Answer from the drawing. Dimensions are ordinates in mm from the lowest x, y and z of the part. Coordinates: 2 decimals unless noted, no trailing zeros. Write each loop counter-clockwise with the first axis right and the second up, starting at its lowest first coordinate (ties: lowest second). Pieces come first, ordered by that corner, then holes. Notation, with made-up numbers: (-37.5, -24.75) -> (19.5, -24.75) arc R18 ccw to (19.5, -10.75) -> close; hole circle Ø7 at (-26, -9.5). An arc over 180 degrees is marked (long way). Return JSON: item names as keys, results as strings.
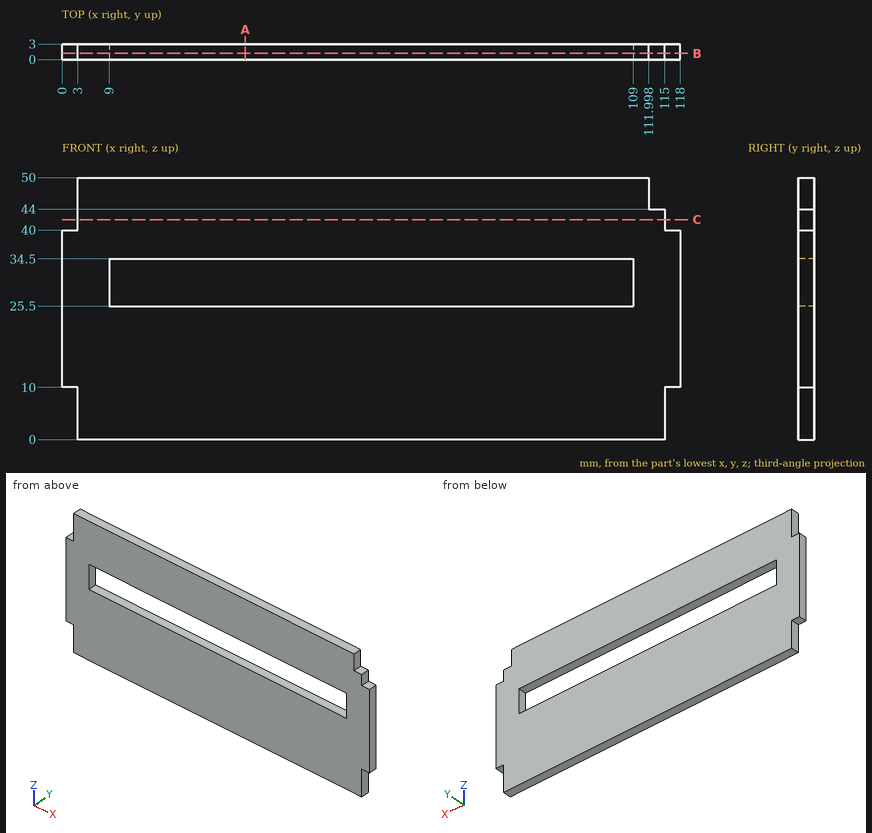
1. Consider L1, parallel to Z at x = 23, y = 2.75; L2, parallel to X at y = 0.25, z = 32. Determine where each line is inside the solid, lowest interval first.
Taken from the geometry:
{"L1": "z = 0 to 25.5, 34.5 to 50", "L2": "x = 0 to 9, 109 to 118"}
2. The part is cut by section C-C (z = 42). Determine the outline of the cut face in (x, y), then the cut area to 3 significant figures.
Taken from the geometry:
{"outline": "(3, 0) -> (115, 0) -> (115, 3) -> (3, 3) -> close", "area": "336 mm2"}
3. Flat-ended cylindrical pins translate along their axes: pin 1 Ø1.5 at (x, y) = (116.5, 1) entering from +Z; pin 2 Ø1.5 at (y, z) = (1, 4.5) entering from -X; pin 3 Ø1.5 at (y, z) = (1, 4) entering from +X. Find the tip coordinate at first contact, or state that the pin passes through.
Taken from the geometry:
{"pin 1": "stops at z = 40", "pin 2": "stops at x = 3", "pin 3": "stops at x = 115"}
4. The part is cut by section A-A (x = 35). Determine the outline of the cut face in (y, z), then the cut area to 3 significant figures.
Taken from the geometry:
{"outline": "(0, 0) -> (3, 0) -> (3, 25.5) -> (0, 25.5) -> close; (0, 34.5) -> (3, 34.5) -> (3, 50) -> (0, 50) -> close", "area": "123 mm2"}
5. The part is cut by section B-B (y = 1.2). Determine the outline of the cut face in (x, z).
Taken from the geometry:
{"outline": "(0, 10) -> (3, 10) -> (3, 0) -> (115, 0) -> (115, 10) -> (118, 10) -> (118, 40) -> (115, 40) -> (115, 44) -> (112, 44) -> (112, 50) -> (3, 50) -> (3, 40) -> (0, 40) -> close; hole (9, 25.5) -> (109, 25.5) -> (109, 34.5) -> (9, 34.5) -> close"}
